Design review of the part built by this model. Coordinates are the model's own, in mm. A direction names the side the tool comes from. Coordinates: 2 decimals unless noted, no trailing zeros. Loops run counter-clockwise (first coordinate to the right, second up) from the corner with the lowest first, then second, coordinate; pieces in that order, holes last. Notation, with made-up numbers: (-39, -26) -> (10, -26) arc R23 cw to (10, 5) -> close; hole circle Ø6 at (-6.5, -8.5). An arc over 180 degrees is marked (long way). One line per item, written item: value. Start each with the question number.
1. Add section C-C on x = 3. Write out the cut boundary in (y, z).
2. Draft analysis for pull direction X (two halves, no side actions). For faces 1 (the cylindrical face through (27.196, 17.972, 10.289)), 2 (the cylindrical face through (-14.94, -19.1, 2.03)), 3 (the flat face through (3, 6, 19.5)), 4 (the cylindrical face through (5.2, -19, 6.1)), state which applies: pulls with the +X half, pulls with the -X half, needs draft (parallel to the pull), parting line crosses it, or undercut.
3. Insertion check: pin 1 (2.5 mm diameter, centred on x = -6.4, y = 11.8, fed in from +Z); pin 2 (3 mm diameter, centred on x = 3, z = 15.5, fed in from -Y); pin 3 (4.5 mm diameter, centred on x = -5, z = 2.5, fed in from +Y). Each pin has a flat end and moves straight along its axis. Give the tip position at first contact, or say it passes through.
4. Add section B-B on x = -6.4. Write out the cut boundary in (y, z), plus the area to 3 significant figures.
5. For probe 1 along X at (y, z) = (11.8, 3); probe 2 along Y at (x, z) = (17, 3.75); probe 3 along Y at (x, z) = (17, 2), list the stretches that pass through material, from the lowest coordinate up.
6. Add section A-A on y = 3.5. Write out the cut boundary in (x, z).
7. Machinability: for faces 5 (the flat face through (15, -19.014, 2.918)), 6 (the flat face through (3, -14, 15)), 7 (the flat face through (-6, 15.3, 2)), which of the approach directions +Z, -Z, +X, -X, +Y, -Y give a long, thin tool a straight path to every point of the face, cutting with its end or side? Answer none if there is none.
8. Add section D-D on z = 4.75. Write out the cut boundary in (x, y), plus the area to 3 significant figures.
```python
from build123d import *

# Parameters (mm, degrees)
PAD_DEPTH       = 12
SKETCH001_R     = 3.7
POCKET_DEPTH    = 5
SKETCH002_R     = 3
POCKET001_DEPTH = 5
POCKET002_DEPTH = 2
SKETCH004_W     = 21.8
SKETCH004_H     = 35.3
SKETCH004_R     = 1
SKETCH004_W_2   = 12.8
SKETCH004_H_2   = 23.3
PAD001_DEPTH    = 4
FILLET_R        = 3
FILLET001_R     = 3
SKETCH005_W     = 6
SKETCH005_H     = 23.3
PAD002_DEPTH    = 13.5
SKETCH006_R     = 1.25
PAD003_DEPTH    = 2
SKETCH007_R     = 1.4
POCKET003_DEPTH = 11
FILLET002_R     = 6
FILLET003_R     = 6
FILLET004_R     = 5.9
FILLET005_R     = 5.9


with BuildPart() as part:
    # Sketch → Pad (new body)
    with BuildSketch(Plane.XY):
        with BuildLine():
            Line((1.5, 20), (29, 20))
            Line((29, 20), (29, 16))
            Line((29, 16), (7.5, 16))
            ThreePointArc((7.5, 16), (6.43934, 15.56066), (6, 14.5))
            Line((6, 14.5), (6, -14.5))
            ThreePointArc((6, -14.5), (6.43934, -15.56066), (7.5, -16))
            Line((7.5, -16), (29, -16))
            Line((29, -16), (29, -20))
            Line((29, -20), (1.5, -20))
            ThreePointArc((0, -18.5), (0.43934, -19.56066), (1.5, -20))
            Line((0, -18.5), (0, 18.5))
            ThreePointArc((1.5, 20), (0.43934, 19.56066), (0, 18.5))
        make_face()
    extrude(amount=PAD_DEPTH)

    # Sketch001 (on Face9 of Pad) → Pocket (cut)
    with BuildSketch(Plane.XZ.offset(20)):
        with Locations((23, 6)):
            Circle(SKETCH001_R)
    extrude(amount=-POCKET_DEPTH, mode=Mode.SUBTRACT)

    # Sketch002 (on Face1 of Pocket) → Pocket001 (cut)
    with BuildSketch(Plane(origin=(0, 20, 0), x_dir=(-1, 0, 0), z_dir=(0, 1, 0))):
        with Locations((-23, 6)):
            Circle(SKETCH002_R)
    extrude(amount=-POCKET001_DEPTH, mode=Mode.SUBTRACT)

    # Sketch003 (on Face14 of Pocket001) → Pocket002 (cut)
    with BuildSketch(Plane.XZ.offset(20)):
        with BuildLine():
            ThreePointArc((7.503922, 8.492299), (5.2, 6), (7.503922, 3.507701))
            Line((7.503922, 3.507701), (22.709804, 2.311398))
            ThreePointArc((22.709804, 2.311398), (26.7, 6), (22.709804, 9.688602))
            Line((22.709804, 9.688602), (7.503922, 8.492299))
        make_face()
    extrude(amount=-POCKET002_DEPTH, mode=Mode.SUBTRACT)

    # Sketch004 (on Face3 of Pocket002) → Pad001 (join)
    with BuildSketch(Plane(origin=(0, 0, 0), x_dir=(1, 0, 0), z_dir=(0, 0, -1))):
        with Locations((-4.9, 2.35)):
            Rectangle(SKETCH004_W, SKETCH004_H)
        with Locations((-6.4, -11.8)):
            Circle(SKETCH004_R, mode=Mode.SUBTRACT)
        with Locations((-6.4, 16.5)):
            Circle(SKETCH004_R, mode=Mode.SUBTRACT)
        with Locations((-6.4, 2.35)):
            Rectangle(SKETCH004_W_2, SKETCH004_H_2, mode=Mode.SUBTRACT)
    extrude(amount=-PAD001_DEPTH)

    # Fillet
    fillet_edges = [part.edges().sort_by_distance(p)[0] for p in [
        (-15.8, -20, 2),
    ]]
    fillet(fillet_edges, radius=FILLET_R)

    # Fillet001
    fillet001_edges = [part.edges().sort_by_distance(p)[0] for p in [
        (-15.8, 15.3, 2),
    ]]
    fillet(fillet001_edges, radius=FILLET001_R)

    # Sketch005 (on Face1 of Fillet001) → Pad002 (join)
    with BuildSketch(Plane.XY.offset(4)):
        with Locations((3, -2.35)):
            Rectangle(SKETCH005_W, SKETCH005_H)
    extrude(amount=PAD002_DEPTH)

    # Sketch006 (on Face47 of Pad002) → Pad003 (join)
    with BuildSketch(Plane.XY.offset(17.5)):
        with Locations((3, 6.15)):
            Circle(SKETCH006_R)
        with Locations((3, -10.85)):
            Circle(SKETCH006_R)
    extrude(amount=PAD003_DEPTH)

    # Sketch007 (on Face47 of Pad003) → Pocket003 (cut)
    with BuildSketch(Plane.XY.offset(17.5)):
        with Locations((3, -2.35)):
            Circle(SKETCH007_R)
    extrude(amount=-POCKET003_DEPTH, mode=Mode.SUBTRACT)

    # Fillet002
    fillet002_edges = [part.edges().sort_by_distance(p)[0] for p in [
        (29, -18, 12),
    ]]
    fillet(fillet002_edges, radius=FILLET002_R)

    # Fillet003
    fillet003_edges = [part.edges().sort_by_distance(p)[0] for p in [
        (29, 18, 12),
    ]]
    fillet(fillet003_edges, radius=FILLET003_R)

    # Fillet004
    fillet004_edges = [part.edges().sort_by_distance(p)[0] for p in [
        (29, -18, 0),
    ]]
    fillet(fillet004_edges, radius=FILLET004_R)

    # Fillet005
    fillet005_edges = [part.edges().sort_by_distance(p)[0] for p in [
        (29, 18, 0),
    ]]
    fillet(fillet005_edges, radius=FILLET005_R)


solid = part.part
```
Worked answers:
1. outline: (-20, 0) -> (20, 0) -> (20, 12) -> (9.3, 12) -> (9.3, 17.5) -> (7.4, 17.5) -> (7.4, 19.5) -> (4.9, 19.5) -> (4.9, 17.5) -> (-0.95, 17.5) -> (-0.95, 6.5) -> (-3.75, 6.5) -> (-3.75, 17.5) -> (-9.6, 17.5) -> (-9.6, 19.5) -> (-12.1, 19.5) -> (-12.1, 17.5) -> (-14, 17.5) -> (-14, 12) -> (-20, 12) -> close
2. face 1: pulls with the +X half
2. face 2: pulls with the -X half
2. face 3: needs draft
2. face 4: undercut
3. pin 1: stops at z = 4
3. pin 2: stops at y = -14
3. pin 3: stops at y = 15.3
4. outline: (-20, 0) -> (-17.5, 0) -> (-17.5, 4) -> (-20, 4) -> close; (-15.5, 0) -> (-14, 0) -> (-14, 4) -> (-15.5, 4) -> close; (9.3, 0) -> (10.8, 0) -> (10.8, 4) -> (9.3, 4) -> close; (12.8, 0) -> (15.3, 0) -> (15.3, 4) -> (12.8, 4) -> close
4. area: 32.0 mm²
5. probe 1: x = -15.8 to -7.4, -5.4 to 6
5. probe 2: y = -18 to -16, 16 to 20
5. probe 3: y = -20 to -16, 16 to 20
6. outline: (-15.8, 0) -> (-12.8, 0) -> (-12.8, 4) -> (-15.8, 4) -> close; (0, 0) -> (6, 0) -> (6, 17.5) -> (0, 17.5) -> close
7. face 5: -Y
7. face 6: +Z, +X, -X, -Y
7. face 7: +Z, -Z, -X, +Y
8. outline: (0, -18.5) arc R1.5 ccw to (1.5, -20) -> (5.53, -20) -> (5.53, -18) -> (19.52, -18) -> (19.52, -16) -> (7.5, -16) arc R1.5 cw to (6, -14.5) -> (6, 14.5) arc R1.5 cw to (7.5, 16) -> (20.27, 16) -> (20.27, 20) -> (1.5, 20) arc R1.5 ccw to (0, 18.5) -> close; (25.73, 16) -> (28.89, 16) -> (28.89, 20) -> (25.73, 20) -> close; (26.48, -20) -> (28.89, -20) -> (28.89, -16) -> (26.48, -16) -> close
8. area: 345 mm²
